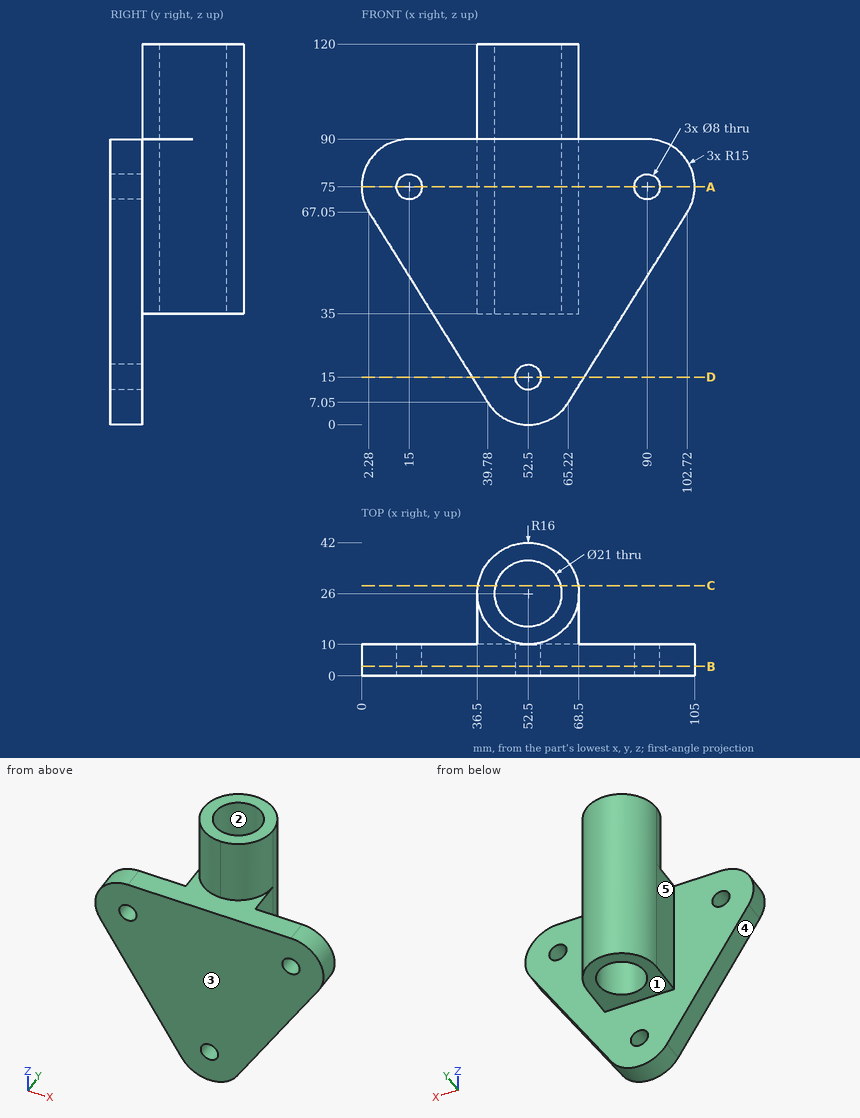
Study the drawing (mm; zero at the part's minimum x, y, z) and answer. A direction names the side the tool comes from. Coordinates: 2 decimals unless noted, no trailing zeros. Order: outer loops, then holes, each group sorted by start corner. A loop starts at its lowest first (then second) coordinate and runs counter-clockwise, first axis right, second up. Notation, with made-up numbers: (7, 64) -> (62, 64) arc R12 ccw to (62, 82) -> close; hole circle Ø6 at (79, 68). An arc over 180 degrees is marked (long way). Answer in a Markdown table with one row per item. Add a question column.
Item 1: Which of the six approach directions +Z, -Z, +X, -X, +Y, -Y give full straight-line access (tool end or side, diameter ignored) to the marked faces 4 and 5?
Item 2: Find section A-A (z = 75). Write down the section's boundary in (x, y).
Item 3: Find section B-B (y = 3). Write down the section's boundary in (x, z).
Item 4: Determine the mould class of the marked faces 1, 2 and 3 for opening direction Y: +Y half, -Y half, draft (parallel to the pull), parting line (faces both ways), or undercut.
Item 5: Find section C-C (y = 28.5). Write down the section's boundary in (x, z).
Item 6: Find section D-D (z = 15). Write down the section's boundary in (x, y), then the cut area to 3 significant figures.
Item 7: Find the intervals of material crossed by L1, parallel to X at y = 5, z = 75; L2, parallel to Y at x = 52.5, z = 73.5; L3, parallel to Y at x = 77, z = 28, in increasing order. Write a range as from..to.
Item 8: Each of these flat-tipped pins is pushed along its axis until it touches: P1, Ø1, axis at x = 57, z = 46, coming from the +Y side; P2, Ø12, axis at y = 24.5, z = 47.5, coming from the +X side; P3, Ø4, axis at y = 37, z = 89.5, coming from the +X side; P4, Ø2, axis at x = 69, z = 31, coming from the -Y side. Where does it stop, or does it pass through?
Result set:
| question | item | result |
|---|---|---|
| 1 | face 4 | -Z, -X, +Y, -Y |
| 1 | face 5 | +Z, -Z, -X, +Y |
| 2 | outline | (0, 0) -> (11, 0) -> (11, 10) -> (0, 10) -> close; (19, 0) -> (86, 0) -> (86, 10) -> (68.5, 10) -> (68.5, 26) arc R16 ccw to (36.5, 26) -> (36.5, 10) -> (19, 10) -> close; (94, 0) -> (105, 0) -> (105, 10) -> (94, 10) -> close; hole circle Ø21 at (52.5, 26) |
| 3 | outline | (2.28, 67.05) -> (39.78, 7.05) arc R15 ccw to (65.22, 7.05) -> (102.72, 67.05) arc R15 ccw to (90, 90) -> (15, 90) arc R15 ccw to start; hole circle Ø8 at (15, 75); hole circle Ø8 at (52.5, 15); hole circle Ø8 at (90, 75) |
| 4 | face 1 | draft |
| 4 | face 2 | undercut |
| 4 | face 3 | -Y half |
| 5 | outline | (36.7, 35) -> (42.3, 35) -> (42.3, 120) -> (36.7, 120) -> close; (62.7, 35) -> (68.3, 35) -> (68.3, 120) -> (62.7, 120) -> close |
| 6 | outline | (34.81, 0) -> (48.5, 0) -> (48.5, 10) -> (34.81, 10) -> close; (56.5, 0) -> (70.19, 0) -> (70.19, 10) -> (56.5, 10) -> close |
| 6 | area | 274 mm² |
| 7 | L1 | x = 0..11, 19..86, 94..105 |
| 7 | L2 | y = 0..15.5, 36.5..42 |
| 7 | L3 | y = 0..10 |
| 8 | P1 | stops at y = 41.49 |
| 8 | P2 | stops at x = 68.5 |
| 8 | P3 | stops at x = 65.73 |
| 8 | P4 | stops at y = 0 |
